Build history of the part. All positions in model axes, mm. A direction names the side the tool comes from. Coordinates: 2 decimals unless noted, no trailing zeros. Loops run counter-clockwise (first coordinate to the right, second up) from the corner with the lowest first, then second, coordinate; pieces in that order, holes last.
Item 1: 3-axis set-ups, long thin cutter, end or side, ignore diameter. For faces 1 (the face through (99.8, 29.6, 2.5)), 2 (the face through (76, 95, 0)): which of +Z, -Z, +X, -X, +Y, -Y reach the whole face in a straight line?
Item 2: Cut at A-A (x = 100). List the corners of the cut face in (y, z).
Item 3: Mould opens along Y. For faces 3 (the face through (99, 130, 5)), 4 (the face through (138.153, 77.015, 6.302)), 5 (the face through (99, 0, 5)) say: released by +Y, released by -Y, zero draft, split by the parting line, or undercut.
Item 4: Cut at B-B (y = 96). List the corners of the cut face in (x, z), and give its area (3 significant figures).
Item 5: Cut at C-C (z = 5.5). Count the separate pieces of the cut face and the enclosed holes in it, and give its area (3 significant figures).
Item 6: Drill centre lines: line 1 along Y through (x, z) = (185, 3.5); line 2 along Y through (x, z) = (155, 6); line 3 along X through (y, z) = (115, 4.75). Where is each one in solid material? Low to high.
from build123d import *

# Parameters (mm, degrees)
SKETCH_W     = 200
SKETCH_H     = 130
SKETCH_R     = 35
SKETCH_R_2   = 1.5
PAD_DEPTH    = 10
SKETCH001_R  = 40
POCKET_DEPTH = 7.5
FILLET_R     = 3


with BuildPart() as part:
    # Sketch → Pad (new body)
    with BuildSketch(Plane.XY):
        with Locations((100, 65)):
            Rectangle(SKETCH_W, SKETCH_H)
        with Locations((100, 65)):
            Circle(SKETCH_R, mode=Mode.SUBTRACT)
        with Locations((45, 115)):
            Circle(SKETCH_R_2, mode=Mode.SUBTRACT)
        with Locations((45, 15)):
            Circle(SKETCH_R_2, mode=Mode.SUBTRACT)
        with Locations((155, 115)):
            Circle(SKETCH_R_2, mode=Mode.SUBTRACT)
        with Locations((155, 15)):
            Circle(SKETCH_R_2, mode=Mode.SUBTRACT)
        with Locations((185, 30)):
            Circle(SKETCH_R_2, mode=Mode.SUBTRACT)
        with Locations((135.353085, 100.338453)):
            Circle(SKETCH_R_2, mode=Mode.SUBTRACT)
        with Locations((64.627773, 29.642413)):
            Circle(SKETCH_R_2, mode=Mode.SUBTRACT)
        with Locations((64.64463, 100.35537)):
            Circle(SKETCH_R_2, mode=Mode.SUBTRACT)
        with Locations((135.352442, 29.63292)):
            Circle(SKETCH_R_2, mode=Mode.SUBTRACT)
        with Locations((175, 20)):
            Circle(SKETCH_R_2, mode=Mode.SUBTRACT)
        with Locations((175, 40)):
            Circle(SKETCH_R_2, mode=Mode.SUBTRACT)
        with Locations((185, 50)):
            Circle(SKETCH_R_2, mode=Mode.SUBTRACT)
        with Locations((175, 90)):
            Circle(SKETCH_R_2, mode=Mode.SUBTRACT)
        with Locations((175, 110)):
            Circle(SKETCH_R_2, mode=Mode.SUBTRACT)
        with Locations((185, 80)):
            Circle(SKETCH_R_2, mode=Mode.SUBTRACT)
        with Locations((185, 100)):
            Circle(SKETCH_R_2, mode=Mode.SUBTRACT)
        with Locations((15, 30)):
            Circle(SKETCH_R_2, mode=Mode.SUBTRACT)
        with Locations((25, 20)):
            Circle(SKETCH_R_2, mode=Mode.SUBTRACT)
        with Locations((25, 40)):
            Circle(SKETCH_R_2, mode=Mode.SUBTRACT)
        with Locations((15, 50)):
            Circle(SKETCH_R_2, mode=Mode.SUBTRACT)
        with Locations((25, 90)):
            Circle(SKETCH_R_2, mode=Mode.SUBTRACT)
        with Locations((25, 110)):
            Circle(SKETCH_R_2, mode=Mode.SUBTRACT)
        with Locations((15, 80)):
            Circle(SKETCH_R_2, mode=Mode.SUBTRACT)
        with Locations((15, 100)):
            Circle(SKETCH_R_2, mode=Mode.SUBTRACT)
    extrude(amount=PAD_DEPTH)

    # Sketch001 (on Face31 of Pad) → Pocket (cut)
    with BuildSketch(Plane.XY.offset(10)):
        with Locations((100, 65)):
            Circle(SKETCH001_R)
    extrude(amount=-POCKET_DEPTH, mode=Mode.SUBTRACT)

    # Fillet
    fillet_edges = [part.edges().sort_by_distance(p)[0] for p in [
        (200, 0, 5),
        (200, 130, 5),
        (0, 0, 5),
        (0, 130, 5),
    ]]
    fillet(fillet_edges, radius=FILLET_R)


solid = part.part
Filled sheet:
1. face 1: +Z
1. face 2: -Z, +X, -X, +Y, -Y
2. outline: (0, 0) - (30, 0) - (30, 2.5) - (25, 2.5) - (25, 10) - (0, 10) - close; (100, 0) - (130, 0) - (130, 10) - (105, 10) - (105, 2.5) - (100, 2.5) - close
3. face 3: released by +Y
3. face 4: undercut
3. face 5: released by -Y
4. outline: (0, 0) - (83.75, 0) - (83.75, 2.5) - (74.72, 2.5) - (74.72, 10) - (0, 10) - close; (116.25, 0) - (200, 0) - (200, 10) - (125.28, 10) - (125.28, 2.5) - (116.25, 2.5) - close
4. area: 1,540 mm2
5. separate pieces: 1
5. enclosed holes: 25
5. area: 20,800 mm2
6. line 1: y = 0 to 28.5, 31.5 to 48.5, 51.5 to 78.5, 81.5 to 98.5, 101.5 to 130
6. line 2: y = 0 to 13.5, 16.5 to 113.5, 116.5 to 130
6. line 3: x = 0 to 43.5, 46.5 to 153.5, 156.5 to 200
